```python
from build123d import *

# Parameters (mm, degrees)
BOSS_EXTRUDE1_DEPTH      = 0.3175
BOSS_EXTRUDE1_DEPTH_BACK = 0.3175
FILLET1_R                = 0.4445
FILLET2_R                = 0.22225


with BuildPart() as part:
    # Sketch3 → Boss-Extrude1 (new body, two sides)
    with BuildSketch(Plane(origin=(0, 0, 0), x_dir=(0, 0, -1), z_dir=(1, 0, 0))) as boss_extrude1_sk:
        with BuildLine():
            Line((2.927731526, -0.975910509), (4.620320242, -1.540106747))
            ThreePointArc((4.620320242, -1.540106747), (2.847682435, -3.950948327), (0, -4.870245161))
            Line((0, -4.870245161), (0, -3.0861))
            ThreePointArc((0, -3.0861), (-0.975910509, -2.927731526), (-1.85166, -2.46888))
            Line((-1.85166, -2.46888), (-5.273248683, -3.537703821))
            ThreePointArc((-5.273248683, -3.537703821), (6.35, 0), (-5.273248683, 3.537703821))
            Line((-5.273248683, 3.537703821), (-1.85166, 2.46888))
            ThreePointArc((-1.85166, 2.46888), (-0.975910509, 2.927731526), (0, 3.0861))
            Line((0, 3.0861), (0, 4.870245161))
            ThreePointArc((0, 4.870245161), (2.847682435, 3.950948327), (4.620320242, 1.540106747))
            Line((4.620320242, 1.540106747), (2.927731526, 0.975910509))
            ThreePointArc((2.927731526, 0.975910509), (3.0861, 0), (2.927731526, -0.975910509))
        make_face()
    extrude(amount=BOSS_EXTRUDE1_DEPTH)
    extrude(boss_extrude1_sk.sketch, amount=-BOSS_EXTRUDE1_DEPTH_BACK)

    # Fillet1
    fillet1_edges = [part.edges().sort_by_distance(p)[0] for p in [
        (0, 1.540106747, -4.620320242),
        (0, 4.870245161, 0),
        (0, 3.537703821, 5.273248683),
        (0, -3.537703821, 5.273248683),
        (0, -4.870245161, 0),
        (0, -1.540106747, -4.620320242),
    ]]
    fillet(fillet1_edges, radius=FILLET1_R)

    # Fillet2
    fillet2_edges = [part.edges().sort_by_distance(p)[0] for p in [
        (0, 0.975910509, -2.927731526),
        (0, 3.0861, 0),
        (0, 2.46888, 1.85166),
        (0, -2.46888, 1.85166),
        (0, -3.0861, 0),
        (0, -0.975910509, -2.927731526),
    ]]
    fillet(fillet2_edges, radius=FILLET2_R)


solid = part.part
```
Design review of the part built by this model. Coordinates are the model's own, in mm. A direction names the side the tool comes from. Give positions to 0.01 mm unless a question says otherwise; leave off trailing zeros. Write each loop counter-clockwise with the first axis right and the second up, starting at its lowest first coordinate (ties: lowest second). Pieces come first, ordered by that corner, then holes.
(1) Add section B-B (x = 0). Give the boundary of the cut face in (y, z).
Checked values:
outline: (-4.85, -0.49) arc R0.44 cw to (-4.4, 0) - (-3.3, 0) arc R0.22 ccw to (-3.08, 0.21) arc R3.09 cw to (-2.53, 1.76) arc R0.22 ccw to (-2.5, 1.96) - (-3.35, 4.67) arc R0.44 ccw to (-4.06, 4.88) arc R6.35 ccw (long way) to (4.06, 4.88) arc R0.44 ccw to (3.35, 4.67) - (2.5, 1.96) arc R0.22 ccw to (2.53, 1.76) arc R3.09 cw to (3.08, 0.21) arc R0.22 ccw to (3.3, 0) - (4.4, 0) arc R0.44 cw to (4.85, -0.49) arc R4.87 cw to (2, -4.44) arc R0.44 cw to (1.39, -4.18) - (1.04, -3.13) arc R0.22 ccw to (0.78, -2.99) arc R3.09 cw to (-0.78, -2.99) arc R0.22 ccw to (-1.04, -3.13) - (-1.39, -4.18) arc R0.44 cw to (-2, -4.44) arc R4.87 cw to start
(2) Add section D-D (z = -1.75). Give the boundary of the cut face in (x, y).
Checked values:
outline: (-0.32, -6.1) - (0.32, -6.1) - (0.32, -4.54) - (-0.32, -4.54) - close; (-0.32, 4.54) - (0.32, 4.54) - (0.32, 6.1) - (-0.32, 6.1) - close
(3) Add section C-C (y = 0). Give the boundary of the cut face in (x, z), and give its area (3 significant figures).
Checked values:
outline: (-0.32, -6.35) - (0.32, -6.35) - (0.32, -3.09) - (-0.32, -3.09) - close
area: 2.07 mm2
(4) Mouldability with a two-part tool opening along Y and no side actions: class faces 1 (the face through (0.004, -0.218, -6.346)), 2 (the face through (0.318, 0, -4)), 3 (the face through (0.004, 2.932, 3.335)), 4 (the face through (0, 3.97, -2.82)) as +Y half, -Y half, draft (parallel to the pull), parting line (faces both ways), or undercut.
Checked values:
face 1: parting line
face 2: draft
face 3: undercut
face 4: undercut
(5) Clearance check with a flat-ended pin moving along its axis: pin 1 Ø6 at (y, z) = (1, 2) entering from -X. State where the tip first meets the part, or that it passes through.
Checked values:
pin 1: stops at x = -0.32
(6) Add section A-A (z = 3.75). Give the boundary of the cut face in (x, y), and give its area (3 significant figures).
Checked values:
outline: (-0.32, -5.12) - (0.32, -5.12) - (0.32, -3.06) - (-0.32, -3.06) - close; (-0.32, 3.06) - (0.32, 3.06) - (0.32, 5.12) - (-0.32, 5.12) - close
area: 2.62 mm2
(7) Wall thickness on line 1 along Y through (x, z) = (0.15, -4.25); line 2 along Y through (x, z) = (0.2, 4.25); line 3 along Y through (x, z) = (-0.2, -4): over which ranges is each line inside the solid? List them lowest first.
Checked values:
line 1: y = -4.72 to -2.38, -1.42 to 1.42, 2.38 to 4.72
line 2: y = -4.72 to -3.22, 3.22 to 4.72
line 3: y = -4.93 to -2.78, -1.33 to 1.33, 2.78 to 4.93
(8) Tool access review of faces 5 (the face through (-0.318, 0, -4)), 6 (the face through (0, -2.92, 3.3)), 7 (the face through (0.004, -3.93, -2.877)): name each direction out of +Z, -Z, +X, -X, +Y, -Y from which nothing blocks a thin tool from reaching the whole face with its end or side.
Checked values:
face 5: +Z, -Z, -X, +Y, -Y
face 6: +Z, +X, -X
face 7: +X, -X
